The model under review builds one solid part; all positions refer to its coordinate system, in mm. A direction names the side the tool comes from. Coordinates: 2 decimals unless noted, no trailing zeros. Order: outer loops, then holes, each group sorted by start corner. A loop starts at its lowest first (then second) coordinate and runs counter-clockwise, first axis right, second up. Notation, with made-up numbers: M 89,-2 L 96,-2 A25 ccw 96,36 Z; hole C -37.75,47 d1. An arc over 180 degrees is marked long. Answer as CSV lines item,"result". Start each with the question number.
Q1. Consider section C-C on y = 20.92. Write out the cut boundary in (x, z), and give its area (3 significant figures).
Q2. Consider section D-D on y = 2. Write out the cut boundary in (x, z).
Q3. For P1, Ø8, axis at x = -10.5, z = 7, coming from the +Y side; P2, Ø5, axis at x = 0, y = 20.92, coming from the -Z side, all flat-tipped, find the tip position at first contact; note any pin that passes through.
Q4. Machinability: for faces 5 (the face through (-19, -13, -1)), 6 (the face through (0, 2, 0)), which of the approach directions +Z, -Z, +X, -X, +Y, -Y give a long, thin tool a straight path to every point of the face, cutting with its end or side? Answer none if there is none.
Q5. Consider section B-B on z = 29. Write out the cut boundary in (x, y).
Q6. Consider section A-A on x = 0. Write out the cut boundary in (y, z), and give its area (3 significant figures).
Q7. Wall thickness on L1, parallel to Z at x = 9.5, y = -32.45; L2, parallel to X at y = -32, z = 14; L3, parallel to Z at x = 13.5, y = -19.5: over which ranges is each line inside the solid? List them lowest first. Write a range as [from, to].
Q8. The part is to be moulded in two halves that separate along Z. For faces 1 (the face through (15.135, -32.465, 16.836)), 2 (the face through (19, -20, -1)), 3 (the face through (-10.822, -32.465, 20.455)), 4 (the face through (0.27, -28.75, 1.29)), say which applies: +Z half, -Z half, draft (parallel to the pull), parting line (faces both ways), or undercut.
Solid Edge part; units mm, degrees
sketch "Sketch1" plane through (0, 0, 0) normal (0, 0, 1) x (1, 0, 0)
  circle A0 centre (0, -18.93) radius 3.2
  circle A1 centre (0, 20.92) radius 3.2
  line L0 (9, 30) -> (-9, 30)
  arc A2 (-19, 20) -> (-9, 30) centre (-9, 20) cw
  line L1 (-19, 20) -> (-19, -30)
  line L2 (-19, -30) -> (19, -30)
  line L3 (19, -30) -> (19, 20)
  arc A3 (9, 30) -> (19, 20) centre (9, 20) cw
extrude "Protrusion1" add sketch "Sketch1" against normal blind 5
sketch "Sketch2" plane through (0, -30, -2.5) normal (0, -1, 0) x (1, 0, 0)
  circle A0 centre (-9.5, 36) radius 6.1
  circle A1 centre (-9.5, 17) radius 6.1
  circle A2 centre (9.5, 17) radius 6.1
  circle A3 centre (9.5, 36) radius 6.1
  line L0 (9.5, 45.5) -> (-9.5, 45.5)
  arc A4 (-9.5, 45.5) -> (-19, 36) centre (-9.5, 36) ccw
  line L1 (-19, 36) -> (-19, 7.5)
  line L2 (-19, 7.5) -> (-19, -2.5)
  line L3 (-19, -2.5) -> (19, -2.5)
  line L4 (19, -2.5) -> (19, 7.5)
  line L5 (19, 7.5) -> (19, 36)
  arc A5 (9.5, 45.5) -> (19, 36) centre (9.5, 36) cw
extrude "Extrusionsausprägung_2" add sketch "Sketch2" along normal blind 5
chamfer "Fase_1" distance 2.54 angle 45 1 edges at (0, -30, 0)
Evaluation:
1,outline,"M -18.96,-5 L -3.2,-5 L -3.2,0 L -18.96,0 Z; M 3.2,-5 L 18.96,-5 L 18.96,0 L 3.2,0 Z"
1,area,"158 mm²"
2,outline,"M -19,-5 L 19,-5 L 19,0 L -19,0 Z"
3,P1,"stops at y = -30"
3,P2,"passes through"
4,face 5,"+Z, -Z, -X, +Y, -Y"
4,face 6,"+Z, +X, -X, +Y"
5,outline,"M -19,-35 L -13.62,-35 L -13.62,-30 L -19,-30 Z; M -5.38,-35 L 5.38,-35 L 5.38,-30 L -5.38,-30 Z; M 13.62,-35 L 19,-35 L 19,-30 L 13.62,-30 Z"
6,outline,"M -35,-5 L -22.13,-5 L -22.13,0 L -27.46,0 L -30,2.54 L -30,43 L -35,43 Z; M -15.73,-5 L 17.72,-5 L 17.72,0 L -15.73,0 Z; M 24.12,-5 L 30,-5 L 30,0 L 24.12,0 Z"
6,area,"479 mm²"
7,L1,"z = [-5, 8.4], [20.6, 27.4], [39.6, 43]"
7,L2,"x = [-19, -15.58], [-3.42, 3.42], [15.58, 19]"
7,L3,"z = [-5, 0]"
8,face 1,"undercut"
8,face 2,"draft"
8,face 3,"undercut"
8,face 4,"+Z half"
